Can you work these out from the model? Positions are in its coordinate system, mm. Round coordinates to 2 decimals unless told otherwise and drop trailing zeros. Loops run counter-clockwise (first coordinate to the right, second up) from the corner with the lowest first, then second, coordinate; pieces in that order, holes last.
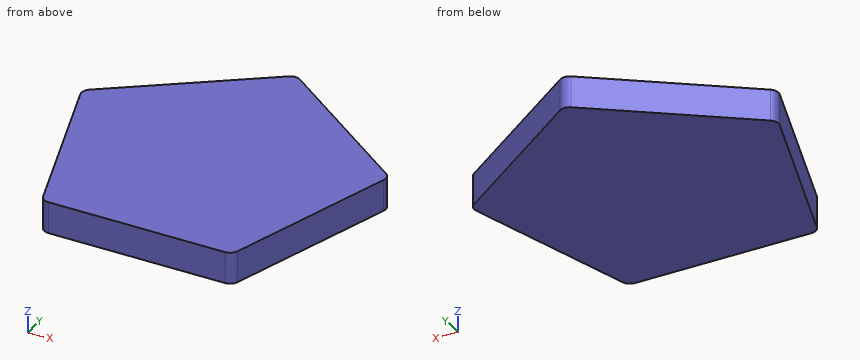
```python
from build123d import *

# Parameters (mm, degrees)
PAD_DEPTH = 10
FILLET_R  = 3


with BuildPart() as part:
    # Sketch → Pad (new body)
    with BuildSketch(Plane.XY):
        Polygon((0, 51.039049), (-48.54102, 15.771933), (-30, -41.291458), (30, -41.291458), (48.54102, 15.771933), align=None)
    extrude(amount=PAD_DEPTH)

    # Fillet
    fillet_edges = [part.edges().sort_by_distance(p)[0] for p in [
        (48.54102, 15.771933, 5),
        (0, 51.039049, 5),
        (-48.54102, 15.771933, 5),
        (-30, -41.291458, 5),
        (30, -41.291458, 5),
    ]]
    fillet(fillet_edges, radius=FILLET_R)


solid = part.part
```
(1) Suppose I cut it at B-B (y = 29). Write out the boundary of the cut face in (x, z), then the cut area to 3 significant figures.
(2) Suppose I cut it at A-A (z = 3). Write out the boundary of the cut face in (x, y), then the cut area to 3 significant figures.
(3) If I drill on line 1 (X direction, y = 14.5, z = 9); line 2 (Y direction, x = 6.5, z = 5.25); line 3 (X direction, y = -4.5, z = 2.25), over which ranges is the centre line in solid material (lowest first)?
(4) For pin 1 (1.5 mm diameter, centred on y = 35, z = 7, fed in from -X); pin 2 (1.5 mm diameter, centred on y = 22, z = 8.5, fed in from -X); pin 3 (1 mm diameter, centred on y = 16.5, z = 3.5, fed in from -X), each with a flat end and sliding along its axis, tell me the tip position at first contact or that it passes through.
(5) Suppose I cut it at C-C (x = -26). Write out the boundary of the cut face in (y, z).
Check result:
1. outline: (-30.33, 0) - (30.33, 0) - (30.33, 10) - (-30.33, 10) - close
1. area: 607 mm2
2. outline: (-47.87, 13.7) - (-30.67, -39.22) arc R3 ccw to (-27.82, -41.29) - (27.82, -41.29) arc R3 ccw to (30.67, -39.22) - (47.87, 13.7) arc R3 ccw to (46.78, 17.05) - (1.76, 49.76) arc R3 ccw to (-1.76, 49.76) - (-46.78, 17.05) arc R3 ccw to start
2. area: 6,190 mm2
3. line 1: x = -48.01 to 48.01
3. line 2: y = -41.29 to 46.32
3. line 3: x = -41.95 to 41.95
4. pin 1: stops at x = -23.11
4. pin 2: stops at x = -41
4. pin 3: stops at x = -47.68
5. outline: (-41.29, 0) - (32.15, 0) - (32.15, 10) - (-41.29, 10) - close
